```python
from build123d import *

# Parameters (mm, degrees)
SKETCH1_W               = 279.4
SKETCH1_H               = 152.4
BOSS_EXTRUDE1_DEPTH     = 12.7
SKETCH2_W               = 25.4
SKETCH2_H               = 12.7
BOSS_EXTRUDE2_DEPTH     = 12.7
LPATTERN1_COUNT         = 5
LPATTERN1_PITCH         = 50.8
MIRROR1_COPY_1_SKETCH_W = 25.4
MIRROR1_COPY_1_SKETCH_H = 12.7
MIRROR1_COPY_1_DEPTH    = 12.7
MIRROR1_COPY_2_SKETCH_W = 25.4
MIRROR1_COPY_2_SKETCH_H = 12.7
MIRROR1_COPY_2_DEPTH    = 12.7
MIRROR1_COPY_3_SKETCH_W = 25.4
MIRROR1_COPY_3_SKETCH_H = 12.7
MIRROR1_COPY_3_DEPTH    = 12.7
MIRROR1_COPY_4_SKETCH_W = 25.4
MIRROR1_COPY_4_SKETCH_H = 12.7
MIRROR1_COPY_4_DEPTH    = 12.7
SKETCH3_W               = 12.7
SKETCH3_H               = 25.4
BOSS_EXTRUDE3_DEPTH     = 12.7
LPATTERN2_COUNT         = 3
LPATTERN2_PITCH         = 50.8
SKETCH4_W               = 25.4
SKETCH4_H               = 12.7
CUT_EXTRUDE1_DEPTH      = 13.7
LPATTERN3_COUNT         = 5
LPATTERN3_PITCH         = 50.8
SKETCH5_W               = 25.4
SKETCH5_H               = 12.7
CUT_EXTRUDE2_DEPTH      = 13.7
LPATTERN4_COUNT         = 5
LPATTERN4_PITCH         = 50.8


with BuildPart() as part:
    # Sketch1 → Boss-Extrude1 (new body)
    with BuildSketch(Plane.XY):
        Rectangle(SKETCH1_W, SKETCH1_H)
    extrude(amount=BOSS_EXTRUDE1_DEPTH)

    # Sketch2 → Boss-Extrude2 (add)
    with BuildSketch(Plane.XZ.offset(76.2)):
        with Locations((-101.6, 6.35)):
            Rectangle(SKETCH2_W, SKETCH2_H)
    boss_extrude2 = extrude(amount=BOSS_EXTRUDE2_DEPTH)

    # LPattern1: Boss-Extrude2 ×5
    with Locations(*[(i * LPATTERN1_PITCH, 0, 0) for i in range(1, LPATTERN1_COUNT)]):
        add(boss_extrude2)

    # Mirror1: Boss-Extrude2 across plane
    add(boss_extrude2.mirror(Plane.ZX))

    # Mirror1 copy 1 sketch → Mirror1 copy 1 (add)
    with BuildSketch(Plane(origin=(50.8, 76.2, 0), x_dir=(1, 0, 0), z_dir=(0, 1, 0))):
        with Locations((-101.6, -6.35)):
            Rectangle(MIRROR1_COPY_1_SKETCH_W, MIRROR1_COPY_1_SKETCH_H)
    extrude(amount=MIRROR1_COPY_1_DEPTH)

    # Mirror1 copy 2 sketch → Mirror1 copy 2 (add)
    with BuildSketch(Plane(origin=(101.6, 76.2, 0), x_dir=(1, 0, 0), z_dir=(0, 1, 0))):
        with Locations((-101.6, -6.35)):
            Rectangle(MIRROR1_COPY_2_SKETCH_W, MIRROR1_COPY_2_SKETCH_H)
    extrude(amount=MIRROR1_COPY_2_DEPTH)

    # Mirror1 copy 3 sketch → Mirror1 copy 3 (add)
    with BuildSketch(Plane(origin=(152.4, 76.2, 0), x_dir=(1, 0, 0), z_dir=(0, 1, 0))):
        with Locations((-101.6, -6.35)):
            Rectangle(MIRROR1_COPY_3_SKETCH_W, MIRROR1_COPY_3_SKETCH_H)
    extrude(amount=MIRROR1_COPY_3_DEPTH)

    # Mirror1 copy 4 sketch → Mirror1 copy 4 (add)
    with BuildSketch(Plane(origin=(203.2, 76.2, 0), x_dir=(1, 0, 0), z_dir=(0, 1, 0))):
        with Locations((-101.6, -6.35)):
            Rectangle(MIRROR1_COPY_4_SKETCH_W, MIRROR1_COPY_4_SKETCH_H)
    extrude(amount=MIRROR1_COPY_4_DEPTH)

    # Sketch3 → Boss-Extrude3 (add)
    with BuildSketch(Plane.ZY.offset(139.7)):
        with Locations((6.35, 63.5)):
            Rectangle(SKETCH3_W, SKETCH3_H)
    boss_extrude3 = extrude(amount=BOSS_EXTRUDE3_DEPTH)

    # LPattern2: Boss-Extrude3 ×3
    with Locations(*[(0, -i * LPATTERN2_PITCH, 0) for i in range(1, LPATTERN2_COUNT)]):
        add(boss_extrude3)

    # Sketch4 → Cut-Extrude1 (cut, through all)
    with BuildSketch(Plane(origin=(0, 0, 0), x_dir=(-1, 0, 0), z_dir=(0, 0, -1))):
        with Locations((-127, 19.05)):
            Rectangle(SKETCH4_W, SKETCH4_H)
    cut_extrude1 = extrude(amount=-CUT_EXTRUDE1_DEPTH, mode=Mode.SUBTRACT)

    # LPattern3: Cut-Extrude1 ×5
    with Locations(*[(-i * LPATTERN3_PITCH, 0, 0) for i in range(1, LPATTERN3_COUNT)]):
        add(cut_extrude1, mode=Mode.SUBTRACT)

    # Sketch5 → Cut-Extrude2 (cut, through all)
    with BuildSketch(Plane.XY.offset(12.7)):
        with Locations((-76.2, 41.275)):
            Rectangle(SKETCH5_W, SKETCH5_H)
    cut_extrude2 = extrude(amount=-CUT_EXTRUDE2_DEPTH, mode=Mode.SUBTRACT)

    # LPattern4: Cut-Extrude2 ×5
    with Locations(*[(i * LPATTERN4_PITCH, 0, 0) for i in range(1, LPATTERN4_COUNT)]):
        add(cut_extrude2, mode=Mode.SUBTRACT)


solid = part.part
```
Read the model definition and answer for the solid it produces. Units are mm, in the model's axes. A direction names the side the tool comes from. Give positions to 0.01 mm unless a question says otherwise; leave off trailing zeros. Order: outer loops, then holes, each group sorted by start corner. A loop starts at its lowest first (then second) coordinate and runs counter-clockwise, first axis right, second up. Notation, with made-up numbers: (-37, 15) -> (-13, 15) arc R7 cw to (-13, 20) -> close; hole circle Ø4 at (26, 59). An arc over 180 degrees is marked (long way). Write item = value, one per line.
1. A cutting plane is placed at C-C, the plane z = 5. Count the separate pieces of the cut face and the enclosed holes in it, and give its area (3 significant figures).
Numbers:
separate_pieces = 1
enclosed_holes = 8
area = 43,500 mm²
2. A cutting plane is placed at D-D, the plane x = -131. Write down the section's boundary in (y, z), and give its area (3 significant figures).
Numbers:
outline = (-76.2, 0) -> (76.2, 0) -> (76.2, 12.7) -> (-76.2, 12.7) -> close
area = 1,940 mm²
3. Given pin 1 (6.5 mm diameter, centred on y = 81, z = 7, fed in from -X); pin 2 (4 mm diameter, centred on x = -70.5, z = 5.5, fed in from +Y); pin 3 (4 mm diameter, centred on x = 79, z = 6.5, fed in from -Y), each flat-ended and moving along its own axis, determine where each tip first touches the part or whether it passes through.
Numbers:
pin_1 = -114.3
pin_2 = 76.2
pin_3 = -76.2
4. The mould has two halves that part along Y. Classify faces 6 (the face through (63.5, -82, 6)), 7 (the face through (-88.9, 41, 6)), 8 (the face through (-26, 76.2, 6)): +Y half, -Y half, draft (parallel to the pull), parting line (faces both ways), or undercut.
Numbers:
face_6 = draft
face_7 = undercut
face_8 = +Y half
5. For faces 1 (the face through (76, 25.4, 6)), 2 (the face through (-63.5, 82, 6)), 3 (the face through (-127, -76.2, 6)), 4 (the face through (-76, -76.2, 6)), 5 (the face through (-146, 50.8, 6)), determine the directions among +Z, -Z, +X, -X, +Y, -Y from which every point of the face is accessible in a straight line to the end or side of a thin tool.
Numbers:
face_1 = +Z, -Z
face_2 = +Z, -Z, +Y
face_3 = +Z, -Z, -X, -Y
face_4 = +Z, -Z, -Y
face_5 = +Z, -Z, -X
6. Straight lines are drawn through the part: line 1 along X through (y, z) = (77, 11); line 2 along Y through (x, z) = (18, 3.5) (3 decimals); line 3 along X through (y, z) = (16, 9.25). For each, find the intervals that lie inside material, in ascending order.
Numbers:
line_1 = -114.3 to -88.9, -63.5 to -38.1, -12.7 to 12.7, 38.1 to 63.5, 88.9 to 114.3
line_2 = -76.2 to 12.7, 25.4 to 34.925, 47.625 to 76.2
line_3 = -152.4 to -88.9, -63.5 to -38.1, -12.7 to 12.7, 38.1 to 63.5, 88.9 to 114.3
7. A cutting plane is placed at A-A, the plane x = -72.5. Write down the section's boundary in (y, z) (3 decimals).
Numbers:
outline = (-76.2, 0) -> (12.7, 0) -> (12.7, 12.7) -> (-76.2, 12.7) -> close; (25.4, 0) -> (34.925, 0) -> (34.925, 12.7) -> (25.4, 12.7) -> close; (47.625, 0) -> (76.2, 0) -> (76.2, 12.7) -> (47.625, 12.7) -> close
8. A cutting plane is placed at B-B, the plane y = 43. Write down the section's boundary in (x, z), and give its area (3 significant figures).
Numbers:
outline = (-139.7, 0) -> (-88.9, 0) -> (-88.9, 12.7) -> (-139.7, 12.7) -> close; (-63.5, 0) -> (-38.1, 0) -> (-38.1, 12.7) -> (-63.5, 12.7) -> close; (-12.7, 0) -> (12.7, 0) -> (12.7, 12.7) -> (-12.7, 12.7) -> close; (38.1, 0) -> (63.5, 0) -> (63.5, 12.7) -> (38.1, 12.7) -> close; (88.9, 0) -> (114.3, 0) -> (114.3, 12.7) -> (88.9, 12.7) -> close
area = 1,940 mm²
